Source: CAD feature listing. Evaluate the final solid. Frame: model axes, mm. A direction names the side the tool comes from. Give positions to 0.01 mm unless a question says otherwise; leave off trailing zeros. Write each loop counter-clockwise with the first axis right and the second up, starting at its lowest first coordinate (ties: lowest second). Pieces come first, ordered by that corner, then holes. Notation, with made-up numbers: (33, -20.75) -> (68, -20.75) arc R29 cw to (68, 2.25) -> close; hole circle Ø3 at (-35.75, -17). An arc over 180 degrees is marked (long way). Use one line per item in the form item = value. Start each with the question number.
(1) Cut plane B-B, the plane x = 0. Output: boundary loops of the cut face in (y, z), and give its area (3 significant figures).
(2) Set-up query: faces 1 (the face through (1.088, 3.014, -0.616)), 2 (the face through (2, -5.013, -1)), 3 (the face through (0, -10.013, 0)). Return all of +Z, -Z, +X, -X, +Y, -Y with unobstructed straight access to the full face (end or side cutting, diameter ignored); none if empty.
(3) First-contact query: P1, Ø1, axis at x = -0.5, y = -5, coming from the +Z side; P2, Ø3, axis at x = 2.5, z = -1, coming from the -Y side; P3, Ø1.5, axis at x = 2.5, z = 1, coming from the -Y side. Flat tips, straight axial feed; report the tip coordinate or a pass-through.
(4) Draft query along Z for faces 4 (the face through (0, 4, 2)), 5 (the face through (1.08, 3.01, 0.63)), 6 (the face through (0.541, -2.542, 2.434)), 7 (the face through (-1.08, 3.01, -0.63)). Return one class per face: pulls with the +Z half, pulls with the -Z half, needs draft (parallel to the pull), parting line crosses it, or undercut.
(5) Material intervals for line 1 along Y through (x, z) = (0.75, 3); line 2 along Y through (x, z) = (2, -1.25); line 3 along Z through (x, y) = (-0.5, 2.75), sorted ascending. Write a range as from..to.
(6) Cut plane A-A, the plane y = 2.75. Output: boundary loops of the cut face in (x, z).
from build123d import *

# Parameters (mm, degrees)
ENL_V_MAT_EXTRU_1_DEPTH = 2


with BuildPart() as part:
    # Esquisse1 → Révolution1 (revolve)
    with BuildSketch(Plane.XY):
        with BuildLine():
            Line((0, 4), (-3.5, 4))
            ThreePointArc((-3.5, 4), (-3.853553391, 3.853553391), (-4, 3.5))
            Line((-4, 3.5), (-4, 0))
            Line((-4, 0), (-2.4935, 0))
            Line((-2.4935, 0), (-2.4935, -5.013))
            Line((-2.4935, -5.013), (-2, -5.013))
            Line((-2, -5.013), (-2, -9.513))
            Line((-2, -9.513), (-1.5, -10.013))
            Line((-1.5, -10.013), (0, -10.013))
            Line((0, -10.013), (0, 4))
        make_face()
    revolve(axis=Axis((0, 15.825722622, 0), (0, -1, 0)))

    # Esquisse2 → Enlèv. mat.-Extru.1 (cut)
    with BuildSketch(Plane(origin=(0, 4, 0), x_dir=(-1, 0, 0), z_dir=(0, 1, 0))):
        Polygon((-1.443375673, 0), (-0.721687836, -1.25), (0.721687836, -1.25), (1.443375673, 0), (0.721687836, 1.25), (-0.721687836, 1.25), align=None)
    extrude(amount=-ENL_V_MAT_EXTRU_1_DEPTH, mode=Mode.SUBTRACT)


solid = part.part
Geometry says:
q1.outline = (-10.01, -1.5) -> (-9.51, -2) -> (-5.01, -2) -> (-5.01, -2.49) -> (0, -2.49) -> (0, -4) -> (3.5, -4) arc R0.5 ccw to (4, -3.5) -> (4, -1.25) -> (2, -1.25) -> (2, 1.25) -> (4, 1.25) -> (4, 3.5) arc R0.5 ccw to (3.5, 4) -> (0, 4) -> (0, 2.49) -> (-5.01, 2.49) -> (-5.01, 2) -> (-9.51, 2) -> (-10.01, 1.5) -> close
q1.area = 71.6 mm^2
q2.face_1 = +Y
q2.face_2 = -Y
q2.face_3 = +Z, -Z, +X, -X, -Y
q3.P1 = 2.49
q3.P2 = -10.01
q3.P3 = -9.57
q4.face_4 = needs draft
q4.face_5 = undercut
q4.face_6 = parting line crosses it
q4.face_7 = undercut
q5.line_1 = 0..4
q5.line_2 = -5.01..4
q5.line_3 = -3.97..-1.25, 1.25..3.97
q6.outline = circle Ø8 at (0, 0); hole (-1.44, 0) -> (-0.72, -1.25) -> (0.72, -1.25) -> (1.44, 0) -> (0.72, 1.25) -> (-0.72, 1.25) -> close
